from build123d import *

# Parameters (mm, degrees)
SKETCH1_W           = 20
SKETCH1_H           = 20
BOSS_EXTRUDE1_DEPTH = 20
CUT_EXTRUDE1_DEPTH  = 25
SKETCH3_W           = 14
SKETCH3_H           = 5
CUT_EXTRUDE2_DEPTH  = 13
FILLET1_R           = 5
FILLET2_R           = 1
FILLET3_R           = 1
SKETCH4_R           = 5.25
BOSS_EXTRUDE2_DEPTH = 5


with BuildPart() as part:
    # Sketch1 → Boss-Extrude1 (new body)
    with BuildSketch(Plane.XY):
        Rectangle(SKETCH1_W, SKETCH1_H)
    extrude(amount=BOSS_EXTRUDE1_DEPTH)

    # Sketch2 → Cut-Extrude1 (cut)
    with BuildSketch(Plane.XY.offset(20)):
        Polygon((4, 2.5), (4, -2.5), (-3, -2.5), (-3, 10), (10, 10), (10, 2.5), align=None)
    extrude(amount=-CUT_EXTRUDE1_DEPTH, mode=Mode.SUBTRACT)

    # Sketch3 → Cut-Extrude2 (cut)
    with BuildSketch(Plane(origin=(10, 0, 0), x_dir=(0, 0, -1), z_dir=(1, 0, 0))):
        with Locations((-7, 0)):
            Rectangle(SKETCH3_W, SKETCH3_H)
    extrude(amount=-CUT_EXTRUDE2_DEPTH, mode=Mode.SUBTRACT)

    # Fillet1
    fillet1_edges = [part.edges().sort_by_distance(p)[0] for p in [
        (10, -10, 10),
        (-10, -10, 10),
    ]]
    fillet(fillet1_edges, radius=FILLET1_R)

    # Fillet2
    fillet2_edges = [part.edges().sort_by_distance(p)[0] for p in [
        (-10, 2.5, 20),
        (-3, 3.75, 0),
        (-3, 3.75, 20),
        (4, 0, 20),
        (4, 0, 14),
        (10, 0, 14),
        (-10, 2.5, 0),
        (10, -1.25, 20),
        (10, -3.75, 0),
        (0, -10, 0),
        (-8.535533906, -8.535533906, 0),
        (8.535533906, -8.535533906, 0),
        (0, -10, 20),
        (-8.535533906, -8.535533906, 20),
        (8.535533906, -8.535533906, 20),
    ]]
    fillet(fillet2_edges, radius=FILLET2_R)

    # Fillet3
    fillet3_edges = [part.edges().sort_by_distance(p)[0] for p in [
        (2.5, -2.5, 0),
        (9.707106781, -2.5, 0.292893219),
        (10, -2.5, 8),
        (9.707106781, 2.5, 19.707106781),
        (10, 2.5, 17),
        (9.707106781, 2.5, 14.292893219),
        (7, 2.5, 14),
        (4.292893219, 2.5, 14.292893219),
        (4, 2.5, 17),
        (4.292893219, 2.5, 19.707106781),
        (7, 2.5, 20),
        (0.5, -2.5, 20),
        (-3.292893219, 10, 0.292893219),
        (-9.707106781, 10, 0.292893219),
        (-6.5, 10, 0),
        (-3, 10, 10),
        (-3.292893219, 10, 19.707106781),
        (-9.707106781, 10, 19.707106781),
        (-6.5, 10, 20),
        (-10, 10, 10),
    ]]
    fillet(fillet3_edges, radius=FILLET3_R)

    # Sketch4 → Boss-Extrude2 (add)
    with BuildSketch(Plane.XZ.offset(10)):
        with Locations(Location((0, 10, 0), (0, 0, 17.752790162))):
            Circle(SKETCH4_R)
    extrude(amount=BOSS_EXTRUDE2_DEPTH)


solid = part.part
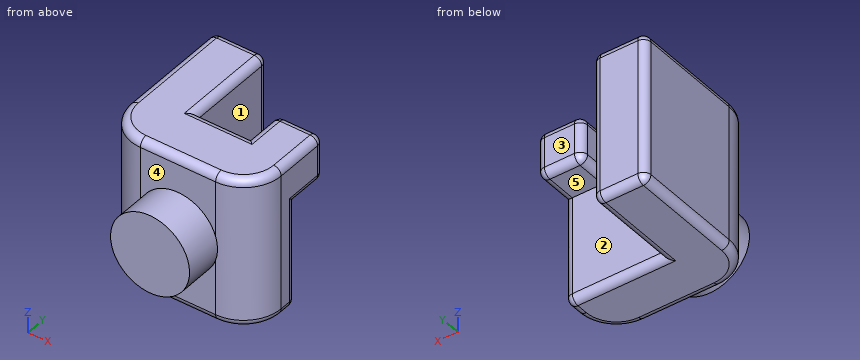
Here's how the part is built. I have some questions about the finished solid (model axes, mm). Face numbers are marked on the shaded views. A direction names the side the tool comes from. Give positions to 0.01 mm unless a question says otherwise; leave off trailing zeros. Order: outer loops, then holes, each group sorted by start corner. A loop starts at its lowest first (then second) coordinate and runs counter-clockwise, first axis right, second up. Notation, with made-up numbers: (26, -33) -> (82, -33) arc R6 ccw to (82, -26) -> close; hole circle Ø4 at (9, 62). An arc over 180 degrees is marked (long way). One line per item, written item: value. Start each with the question number.
1. For the marked faces 1, 2, 3, 4 and 5, which set-ups out of +Z, -Z, +X, -X, +Y, -Y let a thin tool reach every point of the face, with its end or its side?
2. Imagine slicing it at C-C, the plane y = -11.5. List the corners of the cut face in (x, z) for me, plus the area to 3 significant figures.
3. I need wall thicknesses on probe 1 along Z at (x, y) = (5, -2); probe 2 along Y at (x, z) = (1.75, 15.5). Which ranges of each line are inside material? Lowest first, please. Write a range as from..to.
4. Will these pins go through, and if not, where does the flat tip stop? pin 1 Ø12 at (x, z) = (5.5, 14.5) entering from +Y; pin 2 Ø5 at (x, y) = (-2, 4) entering from -Z; pin 3 Ø1 at (y, z) = (-0.5, 8) entering from +X; pin 4 Ø10 at (y, z) = (-12, 16) entering from +X.
5. Imagine slicing it at A-A, the plane x = 0. List the corners of the cut face in (y, z) for me.
Values follow:
1. face 1: +Z, -Z, +Y
1. face 2: -Z, +Y
1. face 3: +Z, -Z, +X, +Y
1. face 4: +Z, -Y
1. face 5: -Z, +X, +Y
2. outline: circle Ø10.5 at (0, 10)
2. area: 86.6 mm2
3. probe 1: z = 14..20
3. probe 2: y = -10..-2.5
4. pin 1: stops at y = 2.5
4. pin 2: stops at z = 0
4. pin 3: stops at x = -3
4. pin 4: stops at x = 9.58
5. outline: (-15, 4.75) -> (-10, 4.75) -> (-10, 1) arc R1 ccw to (-9, 0) -> (-3.5, 0) arc R1 ccw to (-2.5, 1) -> (-2.5, 19) arc R1 ccw to (-3.5, 20) -> (-9, 20) arc R1 ccw to (-10, 19) -> (-10, 15.25) -> (-15, 15.25) -> close
